Part model, mm, in its own coordinate system. A direction names the side the tool comes from. Round coordinates to 2 decimals unless told otherwise and drop trailing zeros. Loops run counter-clockwise (first coordinate to the right, second up) from the corner with the lowest first, then second, coordinate; pieces in that order, holes last.
1) Band-saw the part on C-C, the plane z = -25.4. Write the cut outline in (x, y) (3 decimals), then the cut area to 3 significant figures.
2) Mould opens along Z. For faces 5 (the cylindrical face through (-25.01, -4.83, -11.45)), 6 (the flat face through (7.3, -50.8, 2.3)), 7 (the cylindrical face through (-30.22, -4.83, -3.97)) say: +Z half, -Z half, draft (parallel to the pull), parting line (faces both ways), or undercut.
3) Band-saw the part on D-D, the plane x = 0. State how many separate pieces and enclosed holes the cut face has, then the cut area to 3 significant figures.
4) Probe line 1 (X direction, y = -5.5, z = 12.7); line 2 (X direction, y = -7, z = -12) (3 decimals); line 3 (Y direction, x = 18.5, z = 3.5) (3 decimals). List the from-to ranges inside material, lowest first.
5) Band-saw the part on B-B, the plane y = -14.5. Write the cut outline in (x, z), then the cut area to 3 significant figures.
6) Drop flat-ended pins along their axis: P1, Ø6, axis at x = 21.5, z = -14, coming from the -Y side (3 decimals); P2, Ø1.5, axis at x = -12, y = -29.5, coming from the +Z side; P3, Ø4, axis at x = 0, z = 25.4, coming from the -Y side; P4, Ø1.5, axis at x = 6.5, z = -12.5, coming from the -Y side. Give the stop position or say it passes through.
7) Band-saw the part on A-A, the plane x = -24. Write the cut outline in (y, z) (3 decimals), then the cut area to 3 significant figures.
8) 3-axis set-ups, long thin cutter, end or side, ignore diameter. For faces 1 (the cylindrical face through (13.18, -24.51, -2.93)), 2 (the conical face through (6.368, -6.637, -8.305)), 3 (the cylindrical face through (-10.074, -40.494, -1.323)), 4 (the cylindrical face through (20.5, -4.8, -9.8)): which of +Z, -Z, +X, -X, +Y, -Y reach the whole face in a straight line?
from build123d import *

# Parameters (mm, degrees)
F_1_4_CLEARANCE_HOLE1_D     = 6.5278
F_1_4_CLEARANCE_HOLE1_DEPTH = 22.606
F_1_4_CLEARANCE_HOLE1_TIP   = 1.961148974
CHAMFER1_SIZE               = 1


with BuildPart() as part:
    # Sketch1 → Revolve1 (revolve)
    with BuildSketch(Plane.XY, mode=Mode.PRIVATE) as revolve1_sk:
        Polygon((-7.5, 0), (-30.48, 0), (-30.48, -9.525), (-21, -9.525), (-21, -7.775), (-18, -7.775), (-18, -9.525), (-13.5, -9.525), (-13.5, -38.101219586), (-11, -38.101219586), (-11, -39.688719586), (-10.16, -39.688719586), (-10.16, -41.276219586), (-11.176, -41.276219586), (-11.176, -50.8), (-7.5, -50.8), align=None)
    revolve(revolve1_sk.sketch.rotate(Axis((0, 0, 0), (0, -1, 0)), 270), axis=Axis((0, 0, 0), (0, -1, 0)))

    # Sketch3 → 1/2 NPT Tapped Hole1 (revolve, cut)
    with BuildSketch(Plane(origin=(0, 0, 0), x_dir=(0, 0, 1), z_dir=(1, 0, 0))):
        Polygon((0, 0), (0, 27.970543693), (8.9281, 22.606), (8.9281, 13.462), (10.261665792, 13.462), (10.6647361, 0), align=None)
    revolve(axis=Axis((0, 6.35, 0), (0, -1, 0)), mode=Mode.SUBTRACT)

    # 1/4 Clearance Hole1
    with Locations(Plane(origin=(0, 0, 0), x_dir=(1, 0, 0), z_dir=(0, 1, 0))):
        with Locations((21.997045256, 12.7), (0, 25.4), (-21.997045256, 12.7), (-21.997045256, -12.7), (0, -25.4), (21.997045256, -12.7)):
            Hole(F_1_4_CLEARANCE_HOLE1_D / 2, depth=F_1_4_CLEARANCE_HOLE1_DEPTH)
            with Locations((0, 0, -(F_1_4_CLEARANCE_HOLE1_DEPTH + F_1_4_CLEARANCE_HOLE1_TIP / 2))):  # 118° drill point
                Cone(0, F_1_4_CLEARANCE_HOLE1_D / 2, F_1_4_CLEARANCE_HOLE1_TIP, mode=Mode.SUBTRACT)

    # Chamfer1
    chamfer1_edges = [part.edges().sort_by_distance(p)[0] for p in [
        (0, -9.525, -13.5),
    ]]
    chamfer(chamfer1_edges, length=CHAMFER1_SIZE)


solid = part.part
Reported:
1. outline: (-16.848, -9.525) - (-3.264, -9.525) - (-3.264, 0) - (-16.848, 0) - close; (3.264, -9.525) - (16.848, -9.525) - (16.848, 0) - (3.264, 0) - close
1. area: 259 mm2
2. face 5: undercut
2. face 6: draft
2. face 7: parting line
3. separate pieces: 4
3. enclosed holes: 0
3. area: 629 mm2
4. line 1: x = -27.71 to -25.26, -18.73 to 18.73, 25.26 to 27.71
4. line 2: x = -28.018 to -25.185, -18.809 to 18.809, 25.185 to 28.018
4. line 3: y = -7.775 to 0
5. outline: circle Ø27 at (0, 0); hole circle Ø17.86 at (0, 0)
5. area: 322 mm2
6. P1: stops at y = -9.525
6. P2: stops at z = 7.46
6. P3: passes through
6. P4: stops at y = -38.1
7. outline: (-9.525, -18.789) - (0, -18.789) - (0, -15.277) - (-9.525, -15.277) - close; (-9.525, -10.123) - (0, -10.123) - (0, 10.123) - (-9.525, 10.123) - close; (-9.525, 15.277) - (0, 15.277) - (0, 18.789) - (-9.525, 18.789) - close
7. area: 260 mm2
8. face 1: -Y
8. face 2: +Y
8. face 3: none
8. face 4: +Y, -Y
